Build history of the part. All positions in model axes, mm. A direction names the side the tool comes from. Round coordinates to 2 decimals unless told otherwise and drop trailing zeros. Loops run counter-clockwise (first coordinate to the right, second up) from the corner with the lowest first, then second, coordinate; pieces in that order, holes last.
from build123d import *

# Parameters (mm, degrees)
SKETCH1_W           = 127
SKETCH1_H           = 127
BOSS_EXTRUDE1_DEPTH = 127
SKETCH2_W           = 63.5
SKETCH2_H           = 63.5
CUT_EXTRUDE1_DEPTH  = 128
CHAMFER1_SIZE       = 5.08
FILLET1_R           = 5.08


with BuildPart() as part:
    # Sketch1 → Boss-Extrude1 (new body)
    with BuildSketch(Plane(origin=(0, 0, 0), x_dir=(1, 0, 0), z_dir=(0, 1, 0))):
        Rectangle(SKETCH1_W, SKETCH1_H)
    extrude(amount=BOSS_EXTRUDE1_DEPTH)

    # Sketch2 → Cut-Extrude1 (cut, through all)
    with BuildSketch(Plane(origin=(0, 127, 0), x_dir=(1, 0, 0), z_dir=(0, 1, 0))):
        Rectangle(SKETCH2_W, SKETCH2_H)
    extrude(amount=-CUT_EXTRUDE1_DEPTH, mode=Mode.SUBTRACT)

    # Chamfer1
    chamfer1_edges = [part.edges().sort_by_distance(p)[0] for p in [
        (31.75, 0, 0),
        (0, 0, 31.75),
        (-31.75, 0, 0),
        (0, 0, -31.75),
        (0, 0, 63.5),
        (-63.5, 0, 0),
        (0, 0, -63.5),
        (63.5, 0, 0),
    ]]
    chamfer(chamfer1_edges, length=CHAMFER1_SIZE)

    # Fillet1
    fillet1_edges = [part.edges().sort_by_distance(p)[0] for p in [
        (-63.5, 127, 0),
        (0, 127, 63.5),
        (31.75, 127, 0),
        (0, 127, -31.75),
        (-31.75, 127, 0),
        (0, 127, 31.75),
        (63.5, 127, 0),
        (0, 127, -63.5),
    ]]
    fillet(fillet1_edges, radius=FILLET1_R)


solid = part.part
(1) Slice it at B-B on x = -23. List the corners of the cut face in (y, z).
Responses:
outline: (0, -58.42) - (5.08, -63.5) - (121.92, -63.5) arc R5.08 ccw to (127, -58.42) - (127, -36.83) arc R5.08 ccw to (121.92, -31.75) - (5.08, -31.75) - (0, -36.83) - close; (0, 36.83) - (5.08, 31.75) - (121.92, 31.75) arc R5.08 ccw to (127, 36.83) - (127, 58.42) arc R5.08 ccw to (121.92, 63.5) - (5.08, 63.5) - (0, 58.42) - close
(2) Pull direction Z, two halves, no side cores. Call faces 5 (the face through (0.889, 125.551, -61.972)), 6 (the face through (-0.52, 2.58, 34.25)), 7 (the face through (-33.278, 125.551, -0.516)), 8 (the face through (-63.5, 63, 1)): +Z half, -Z half, draft (parallel to the pull), parting line (faces both ways), or undercut.
Responses:
face 5: -Z half
face 6: undercut
face 7: undercut
face 8: draft
(3) Slice it at C-C on y = 84. List the corners of the cut face in (x, z), plus the area to 3 significant figures.
Responses:
outline: (-63.5, -63.5) - (63.5, -63.5) - (63.5, 63.5) - (-63.5, 63.5) - close; hole (-31.75, -31.75) - (31.75, -31.75) - (31.75, 31.75) - (-31.75, 31.75) - close
area: 12,100 mm2
(4) Probe line 1 (Z direction, x = -24, y = 27). List the from-to ranges inside material, lowest first.
Responses:
line 1: z = -63.5 to -31.75, 31.75 to 63.5
(5) Slice it at A-A on z = 12. List the corners of the cut face in (x, y).
Responses:
outline: (-63.5, 5.08) - (-58.42, 0) - (-36.83, 0) - (-31.75, 5.08) - (-31.75, 121.92) arc R5.08 ccw to (-36.83, 127) - (-58.42, 127) arc R5.08 ccw to (-63.5, 121.92) - close; (31.75, 5.08) - (36.83, 0) - (58.42, 0) - (63.5, 5.08) - (63.5, 121.92) arc R5.08 ccw to (58.42, 127) - (36.83, 127) arc R5.08 ccw to (31.75, 121.92) - close
(6) Which spindle directions (+Z, -Z, +X, -X, +Y, -Y) get a long thin tool onto all of the face, cutting with end or side? Do faces 1 (the face through (0.516, 125.551, 33.278)), 2 (the face through (0, 64, -31.75)), 3 (the face through (-1, 63, 63.5)), 4 (the face through (-34.25, 2.58, 0.52)). Say none if no direction does.
Responses:
face 1: +Y
face 2: +Y, -Y
face 3: +Z, +X, -X, +Y, -Y
face 4: -Y
